```python
from build123d import *

# Parameters (mm, degrees)
F0_R     = 32.5
F0_R_2   = 27.78
F1_DEPTH = 5
F0_R_3   = 1.35
F0_R_4   = 20.03
F2_DEPTH = 12
F3_DEPTH = 6


with BuildPart() as f1:
    # F0 (on Top) → F1 (new body)
    with BuildSketch(Plane.XY):
        Circle(F0_R)
        Circle(F0_R_2, mode=Mode.SUBTRACT)
    extrude(amount=F1_DEPTH)

    # F0 (on Top) → F2 (join)
    with BuildSketch(Plane.XY):
        Circle(F0_R_2)
        with Locations((0, -23.905)):
            Circle(F0_R_3, mode=Mode.SUBTRACT)
        with Locations((-23.905, 0)):
            Circle(F0_R_3, mode=Mode.SUBTRACT)
        Circle(F0_R_4, mode=Mode.SUBTRACT)
        with Locations((23.905, 0)):
            Circle(F0_R_3, mode=Mode.SUBTRACT)
        with Locations((0, 23.905)):
            Circle(F0_R_3, mode=Mode.SUBTRACT)
    extrude(amount=F2_DEPTH)

    # F0 (on Top) → F3 (join)
    with BuildSketch(Plane.XY):
        with Locations((-23.905, 0)):
            Circle(F0_R_3)
        with Locations((0, 23.905)):
            Circle(F0_R_3)
        with Locations((23.905, 0)):
            Circle(F0_R_3)
        with Locations((0, -23.905)):
            Circle(F0_R_3)
    extrude(amount=F3_DEPTH)


solid = f1.part
```
Input: part model. Units: mm. Frame: model coordinates. A direction names the side the tool comes from. Round coordinates to 2 decimals unless told otherwise and drop trailing zeros. Order: outer loops, then holes, each group sorted by start corner. A loop starts at its lowest first (then second) coordinate and runs counter-clockwise, first axis right, second up. Notation, with made-up numbers: (-1.5, 60) - (24.5, 60) arc R18 ccw to (24.5, 93) - close; hole circle Ø11 at (65, 42). An arc over 180 degrees is marked (long way). One line per question, with ' | ' between items. Start each with the question number.
1) Contact query for flat-ended pins moving along their axis: P1, Ø1.4, axis at x = 0, y = 24.5, coming from the +Z side; P2, Ø2.5, axis at x = 0, y = 23.905, coming from the -Z side; P3, Ø4, axis at y = 6, z = 10.5, coming from the +X side; P4, Ø3, axis at y = -23, z = 8, coming from the -X side. Output: stop coordinate, or through.
2) Cut plane A-A, the plane x = 0. Return the cut outline in (y, z) (3 decimals).
3) Ray query, probe 1 along Y at (x, z) = (0, 8.2) (3 decimals); probe 2 along X at (y, z) = (-0.5, 5.5); probe 3 along Y at (x, z) = (-14, 4.5). Return the intervals inside material, ascending.
4) Pull-direction query (Y, two-part tool) for faces 1 (the cylindrical face through (31, 9.76, 2.46)), 2 (the flat face through (14, 15, 0)), 3 (the flat face through (24, 0, 6)); classes: +Y half, -Y half, draft (parallel to the pull), parting line (faces both ways), or undercut.
5) Cut plane D-D, the plane z = 9. Return the cut outline in (x, y) (3 decimals), then the cut area to 3 significant figures.
6) Set-up query: faces 4 (the flat face through (0, -24, 6)), 5 (the cylindrical face through (-4.342, -19.554, 5.916)). Return all of +Z, -Z, +X, -X, +Y, -Y with unobstructed straight access to the full face (end or side cutting, diameter ignored); none if empty.
7) Cut plane C-C, the plane z = 3. Return the cut outline in (x, y).
Worked out:
1) P1: stops at z = 6 | P2: stops at z = 0 | P3: stops at x = 27.49 | P4: stops at x = -17.59
2) outline: (-32.5, 0) - (-20.03, 0) - (-20.03, 12) - (-22.555, 12) - (-22.555, 6) - (-25.255, 6) - (-25.255, 12) - (-27.78, 12) - (-27.78, 5) - (-32.5, 5) - close; (20.03, 0) - (32.5, 0) - (32.5, 5) - (27.78, 5) - (27.78, 12) - (25.255, 12) - (25.255, 6) - (22.555, 6) - (22.555, 12) - (20.03, 12) - close
3) probe 1: y = -27.78 to -25.255, -22.555 to -20.03, 20.03 to 22.555, 25.255 to 27.78 | probe 2: x = -27.78 to -20.02, 20.02 to 27.78 | probe 3: y = -29.33 to -14.32, 14.32 to 29.33
4) face 1: parting line | face 2: draft | face 3: undercut
5) outline: circle Ø55.56 at (0, 0); hole circle Ø2.7 at (-23.905, 0); hole circle Ø40.06 at (0, 0); hole circle Ø2.7 at (0, -23.905); hole circle Ø2.7 at (0, 23.905); hole circle Ø2.7 at (23.905, 0) | area: 1,140 mm^2
6) face 4: +Z | face 5: +Z, -Z
7) outline: circle Ø65 at (0, 0); hole circle Ø40.06 at (0, 0)
